Design review of the part built by this model. Coordinates are the model's own, in mm. Face numbers are marked on the shaded views. Give positions to 0.01 mm unless a question says otherwise; leave off trailing zeros. Loops run counter-clockwise (first coordinate to the right, second up) from the corner with the lowest first, then second, coordinate; pieces in that order, holes last. Notation, with made-up numbers: (81.5, 69) -> (130.5, 69) arc R23 cw to (130.5, 102) -> close; hole circle Ø1 at (13, -10). An arc over 180 degrees is marked (long way). Use a Markdown table: item, result. Add a question column.
1. Add section A-A (z = 0). State the section outline as (x, y) points.
2. Add section D-D (z = -9.75). State the section outline as (x, y) points.
3. Draft analysis for pull direction X (two halves, no side actions). For the marked faces 1, 2 and 3, state which applies: pulls with the +X half, pulls with the -X half, needs draft (parallel to the pull), parting line crosses it, or undercut.
4. Add section C-C (y = 0.5). Count the separate pieces of the cut face and the enclosed holes in it, and give its area (3 significant figures).
5. To check wall thickness, follow line 1 (X direction, y = 1.3, z = 0); line 2 (X direction, y = 0.3, z = -8); line 3 (Z direction, x = 6, y = 0.7). State the ranges of each line that lie inside material, in increasing order.
6. For pin 1 Ø2.5 at (x, z) = (9, 0) entering from -Y; pin 2 Ø1 at (y, z) = (1.5, -1.5) entering from +X; pin 3 Ø1 at (y, z) = (1, 4.5) entering from -X; pin 4 Ø1 at (x, y) = (8.5, 1) entering from -Z, all flat-tipped, find the tip position at first contact; note any pin that passes through.
7. Add section B-B (x = 0). State the section outline as (y, z) points, and give its area (3 significant figures).
```python
from build123d import *

# Parameters (mm, degrees)
SKETCH1_R           = 13.5
BOSS_EXTRUDE1_DEPTH = 2
SKETCH4_R           = 1.5
CUT_EXTRUDE1_DEPTH  = 20.19635382
CIRPATTERN1_COUNT   = 4
SKETCH2_R           = 2
CUT_EXTRUDE2_DEPTH  = 20.19635382


with BuildPart() as part:
    # Sketch1 → Boss-Extrude1 (new body)
    with BuildSketch(Plane(origin=(0, 0, 0), x_dir=(1, 0, 0), z_dir=(0, 1, 0))):
        with Locations(Location((0, 0, 0), (0, 0, 270))):
            Circle(SKETCH1_R)
    extrude(amount=BOSS_EXTRUDE1_DEPTH)

    # Sketch4 → Cut-Extrude1 (cut, through all)
    with BuildSketch(Plane.XZ):
        with Locations(Location((-9, 0, 0), (0, 0, 270))):
            Circle(SKETCH4_R)
        with Locations(Location((-7.071067812, -7.071067812, 0), (0, 0, 270))):
            Circle(SKETCH4_R)
    cut_extrude1 = extrude(amount=-CUT_EXTRUDE1_DEPTH, mode=Mode.SUBTRACT)

    # CirPattern1: Cut-Extrude1 ×4 about axis
    cirpattern1_axis = Axis((0, 0, 0), (0, 1, 0))
    for i in range(1, CIRPATTERN1_COUNT):
        add(cut_extrude1.rotate(cirpattern1_axis, i * 360 / CIRPATTERN1_COUNT), mode=Mode.SUBTRACT)

    # Sketch2 → Cut-Extrude2 (cut, through all)
    with BuildSketch(Plane(origin=(0, 2, 0), x_dir=(1, 0, 0), z_dir=(0, 1, 0))):
        with Locations(Location((0, 0, 0), (0, 0, 270))):
            Circle(SKETCH2_R)
    extrude(amount=-CUT_EXTRUDE2_DEPTH, mode=Mode.SUBTRACT)


solid = part.part
```
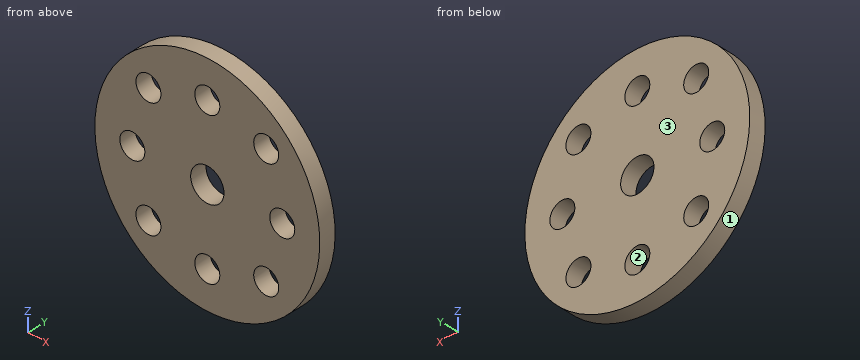
Taken from the geometry:
| question | item | result |
|---|---|---|
| 1 | outline | (-13.5, 0) -> (-10.5, 0) -> (-10.5, 2) -> (-13.5, 2) -> close; (-7.5, 0) -> (-2, 0) -> (-2, 2) -> (-7.5, 2) -> close; (2, 0) -> (7.5, 0) -> (7.5, 2) -> (2, 2) -> close; (10.5, 0) -> (13.5, 0) -> (13.5, 2) -> (10.5, 2) -> close |
| 2 | outline | (-9.34, 0) -> (-1.3, 0) -> (-1.3, 2) -> (-9.34, 2) -> close; (1.3, 0) -> (9.34, 0) -> (9.34, 2) -> (1.3, 2) -> close |
| 3 | face 1 | parting line crosses it |
| 3 | face 2 | undercut |
| 3 | face 3 | needs draft |
| 4 | separate pieces | 1 |
| 4 | enclosed holes | 9 |
| 4 | area | 503 mm^2 |
| 5 | line 1 | x = -13.5 to -10.5, -7.5 to -2, 2 to 7.5, 10.5 to 13.5 |
| 5 | line 2 | x = -10.87 to -8.25, -5.89 to -1.12, 1.12 to 5.89, 8.25 to 10.87 |
| 5 | line 3 | z = -12.09 to -8.12, -6.02 to 6.02, 8.12 to 12.09 |
| 6 | pin 1 | passes through |
| 6 | pin 2 | stops at x = 13.46 |
| 6 | pin 3 | stops at x = -12.89 |
| 6 | pin 4 | stops at z = -10.87 |
| 7 | outline | (0, -13.5) -> (2, -13.5) -> (2, -10.5) -> (0, -10.5) -> close; (0, -7.5) -> (2, -7.5) -> (2, -2) -> (0, -2) -> close; (0, 2) -> (2, 2) -> (2, 7.5) -> (0, 7.5) -> close; (0, 10.5) -> (2, 10.5) -> (2, 13.5) -> (0, 13.5) -> close |
| 7 | area | 34.0 mm^2 |
